Part print with two shaded views. Sizes in mm from the minimum x, y, z corner. A direction names the side the tool comes from. Round coordinates to 2 decimals unless told otherwise and drop trailing zeros. Order: outer loops, then holes, each group sorted by start corner. A loop starts at its lowest first (then second) coordinate and runs counter-clockwise, first axis right, second up. Notation, with made-up numbers: (63, 22) -> (101, 22) arc R21 cw to (101, 40) -> close; hole circle Ø6 at (-5, -12.75). An arc over 180 degrees is marked (long way). Put each result on its own line as item: value. Start each with the question number.
Q1. Cut at C-C, the plane z = 7.5. State how many separate pieces and enclosed holes the cut face has, and give its area (3 significant figures).
Q2. Pull direction X, two halves, no side cores. Call the marked faces 3, 4 and 5: released by +X, released by -X, zero draft, split by the parting line, or undercut.
Q3. Cut at B-B, the plane y = 13.75. List the corners of the cut face in (x, z).
Q4. Cut at A-A, the plane y = 16.25. List the corners of the cut face in (x, z), and give its area (3 significant figures).
Q5. 3-axis set-ups, long thin cutter, end or side, ignore diameter. For the marked faces 1 and 2: which of +Z, -Z, +X, -X, +Y, -Y reach the whole face in a straight line?
Q6. Flat gauge pin, fed straight in: P1, Ø4, axis at y = 12.5, z = 7.5, coming from the +X side. Where does the tip first touch, or does it go through?
Q7. Cut at D-D, the plane x = 20.5. List the corners of the cut face in (y, z), and give its area (3 significant figures).
Q8. Probe L1, parallel to X at y = 13.5, z = 14; L2, parallel to Z at x = 38.5, y = 12.5; L3, parallel to X at y = 17, z = 7.5. List the from-to ranges inside material, lowest first.
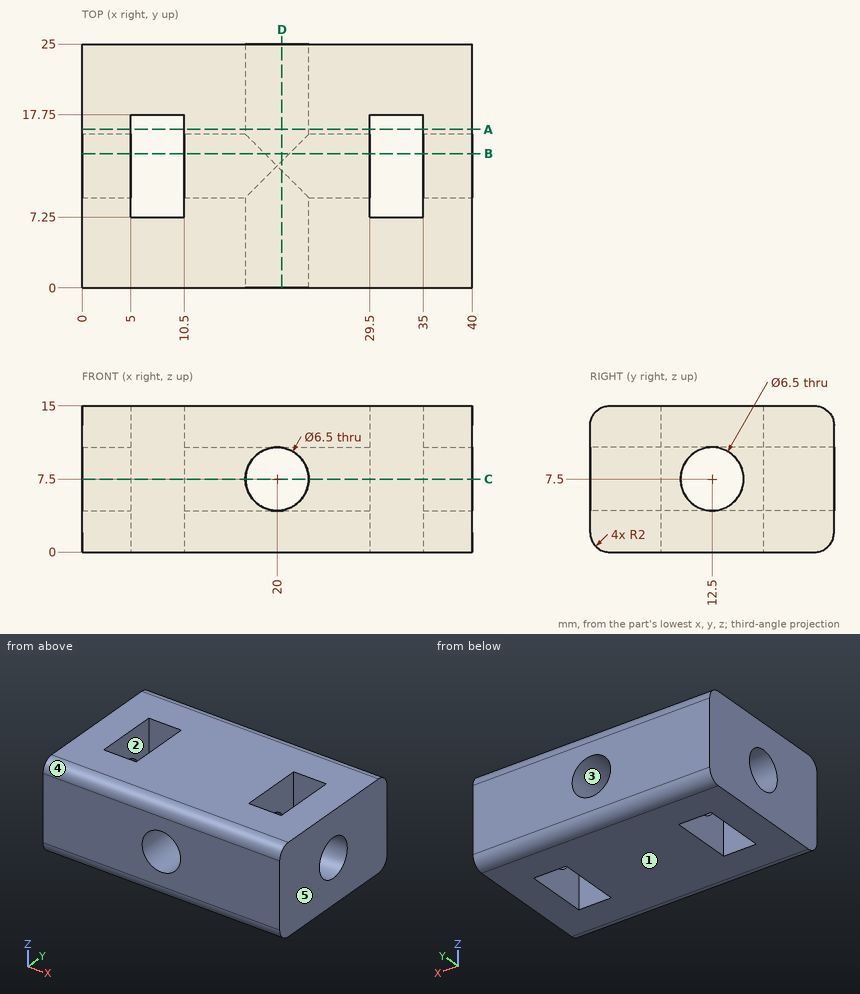
Ans:
1. separate pieces: 4
1. enclosed holes: 0
1. area: 576 mm^2
2. face 3: undercut
2. face 4: zero draft
2. face 5: released by +X
3. outline: (0, 0) -> (5, 0) -> (5, 4.5) -> (0, 4.5) -> close; (0, 10.5) -> (5, 10.5) -> (5, 15) -> (0, 15) -> close; (10.5, 0) -> (29.5, 0) -> (29.5, 4.5) -> (21.25, 4.5) arc R3.25 cw to (18.75, 4.5) -> (10.5, 4.5) -> close; (10.5, 10.5) -> (18.75, 10.5) arc R3.25 cw to (21.25, 10.5) -> (29.5, 10.5) -> (29.5, 15) -> (10.5, 15) -> close; (35, 0) -> (40, 0) -> (40, 4.5) -> (35, 4.5) -> close; (35, 10.5) -> (40, 10.5) -> (40, 15) -> (35, 15) -> close
4. outline: (0, 0) -> (5, 0) -> (5, 15) -> (0, 15) -> close; (10.5, 0) -> (29.5, 0) -> (29.5, 15) -> (10.5, 15) -> close; (35, 0) -> (40, 0) -> (40, 15) -> (35, 15) -> close; hole circle Ø6.5 at (20, 7.5)
4. area: 402 mm^2
5. face 1: -Z, +X, -X, +Y, -Y
5. face 2: +Z, -Z
6. P1: passes through
7. outline: (0, 2) arc R2 ccw to (2, 0) -> (23, 0) arc R2 ccw to (25, 2) -> (25, 4.29) -> (13, 4.29) arc R3.25 cw to (12, 4.29) -> (0, 4.29) -> close; (0, 10.71) -> (12, 10.71) arc R3.25 cw to (13, 10.71) -> (25, 10.71) -> (25, 13) arc R2 ccw to (23, 15) -> (2, 15) arc R2 ccw to (0, 13) -> close
7. area: 211 mm^2
8. L1: x = 0 to 5, 10.5 to 29.5, 35 to 40
8. L2: z = 0 to 4.25, 10.75 to 15
8. L3: x = 0 to 5, 10.5 to 16.75, 23.25 to 29.5, 35 to 40
